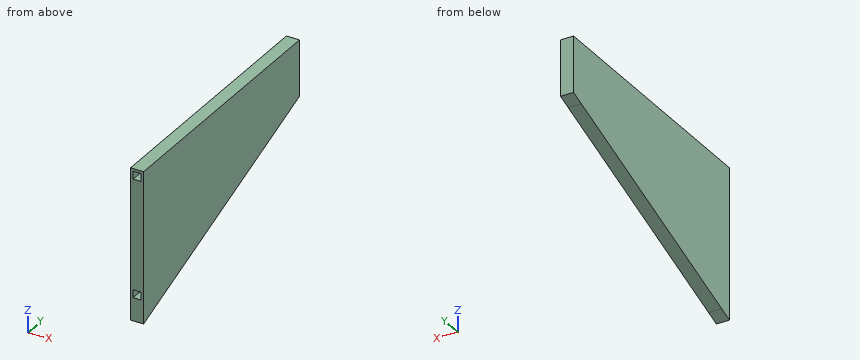
```python
from build123d import *

# Parameters (mm, degrees)
SKETCH1_W           = 100
SKETCH1_H           = 100
BOSS_EXTRUDE1_DEPTH = 10
CUT_EXTRUDE2_DEPTH  = 5
CUT_EXTRUDE4_DEPTH  = 10
CUT_EXTRUDE5_DEPTH  = 5
SKETCH8_W           = 3
SKETCH8_H           = 3
CUT_EXTRUDE6_DEPTH  = 5


with BuildPart() as part:
    # Sketch1 → Boss-Extrude1 (new body)
    with BuildSketch(Plane(origin=(0, 0, 0), x_dir=(0, 0, -1), z_dir=(1, 0, 0))):
        Rectangle(SKETCH1_W, SKETCH1_H)
    extrude(amount=BOSS_EXTRUDE1_DEPTH)

    # Sketch2 → Cut-Extrude2 (cut)
    with BuildSketch(Plane.ZY):
        Polygon((36.397023427, 50), (33.897023427, 50), (-0.680148829, -45), (4.319851171, -45), (38.897023427, 50), align=None)
    extrude(amount=-CUT_EXTRUDE2_DEPTH, mode=Mode.SUBTRACT)

    # Sketch5 → Cut-Extrude4 (cut)
    with BuildSketch(Plane.ZY):
        Polygon((28.576134564, 50), (-50, 50), (-50, -50), (-7.820888862, -50), (-6.001037691, -45), (26.756283393, 45), align=None)
    extrude(amount=-CUT_EXTRUDE4_DEPTH, mode=Mode.SUBTRACT)

    # Sketch7 → Cut-Extrude5 (cut)
    with BuildSketch(Plane.ZY):
        Polygon((28.576134564, 50), (50, 50), (50, -50), (-7.820888862, -50), align=None)
    extrude(amount=-CUT_EXTRUDE5_DEPTH, mode=Mode.SUBTRACT)

    # Sketch8 → Cut-Extrude6 (cut)
    with BuildSketch(Plane.XZ.offset(50)):
        with Locations((7.5, 47.5)):
            Rectangle(SKETCH8_W, SKETCH8_H)
        with Locations((7.5, 2.5)):
            Rectangle(SKETCH8_W, SKETCH8_H)
    extrude(amount=-CUT_EXTRUDE6_DEPTH, mode=Mode.SUBTRACT)


solid = part.part
```
Can you work these out from the model? Positions are in its coordinate system, mm. Coordinates: 2 decimals unless noted, no trailing zeros. Loops run counter-clockwise (first coordinate to the right, second up) from the corner with the lowest first, then second, coordinate; pieces in that order, holes last. Notation, with made-up numbers: M 12.5,-18.5 L 31.5,-18.5 A26 ccw 31.5,20.5 Z; hole C -16.75,11 d2. An arc over 180 degrees is marked long. Put each result on its own line as item: value. Start each with the question number.
(1) Imagine slicing it at A-A on x = 7.65. List the corners of the cut face in (y, z) for me.
(2) Imagine slicing it at C-C on z = 9. List the corners of the cut face in (x, y) for me, and give its area (3 significant figures).
(3) Imagine slicing it at B-B on y = 9.5. List the corners of the cut face in (x, z) for me, and give its area (3 significant figures).
(4) Will these pins go through, and if not, where does the flat tip stop? pin 1 Ø1.5 at (x, z) = (8, 2.5) entering from -Y; pin 2 Ø2 at (x, y) = (7, 12) entering from -Z; pin 3 Ø2.5 at (x, y) = (8, -46.5) entering from -Z.
(5) I need wall thicknesses on probe 1 along Z at (x, y) = (7.5, 14); probe 2 along Z at (x, y) = (5.75, -42). Which ranges of each line are inside material? Lowest first, please.
Worked answers:
1. outline: M -50,-7.82 L 50,28.58 L 50,50 L -50,50 L -50,49 L -45,49 L -45,46 L -50,46 L -50,4 L -45,4 L -45,1 L -50,1 Z
2. outline: M 5,-50 L 10,-50 L 10,-3.78 L 5,-3.78 Z
2. area: 231 mm2
3. outline: M 5,13.84 L 10,13.84 L 10,50 L 5,50 Z
3. area: 181 mm2
4. pin 1: stops at y = -45
4. pin 2: stops at z = 14.38
4. pin 3: stops at z = -7
5. probe 1: z = 15.47 to 50
5. probe 2: z = -4.91 to 50
